```python
from build123d import *

# Parameters (mm, degrees)
BOSS_EXTRUDE1_DEPTH = 3.175
FILLET1_R           = 3.175


with BuildPart() as part:
    # Sketch1 → Boss-Extrude1 (new body)
    with BuildSketch(Plane.XY):
        with BuildLine():
            Line((0, 0), (3.175, 0))
            Line((3.175, 0), (3.175, 6.35))
            Line((3.175, 6.35), (0, 6.35))
            Line((0, 6.35), (0, 12.7))
            Line((0, 12.7), (3.175, 12.7))
            Line((3.175, 12.7), (3.175, 19.05))
            Line((3.175, 19.05), (0, 19.05))
            Line((0, 19.05), (-6.35, 19.05))
            ThreePointArc((-6.35, 19.05), (-9.044076836, 20.165923164), (-10.16, 22.86))
            Line((-10.16, 22.86), (-10.16, 50.8))
            Line((-10.16, 50.8), (-22.86, 50.8))
            Line((-22.86, 50.8), (-22.86, 16.51))
            ThreePointArc((-22.86, 16.51), (-18.024332957, 4.835667043), (-6.35, 0))
            Line((-6.35, 0), (0, 0))
        make_face()
    extrude(amount=BOSS_EXTRUDE1_DEPTH)

    # Fillet1
    fillet1_edges = [part.edges().sort_by_distance(p)[0] for p in [
        (-22.86, 50.8, 1.5875),
        (-10.16, 50.8, 1.5875),
    ]]
    fillet(fillet1_edges, radius=FILLET1_R)


solid = part.part
```
Source: CAD feature listing. Evaluate the final solid. Frame: model axes, mm. A direction names the side the tool comes from. Round coordinates to 2 decimals unless told otherwise and drop trailing zeros. Loops run counter-clockwise (first coordinate to the right, second up) from the corner with the lowest first, then second, coordinate; pieces in that order, holes last. Notation, with made-up numbers: M 16.5,14.25 L 65.5,14.25 A31 cw 65.5,41.25 Z; hole C 27.25,43.25 d10. An arc over 180 degrees is marked long. Use a Markdown table: item, result. Add a question column.
1. Cut plane C-C, the plane x = -3.5. Output: boundary loops of the cut face in (y, z) (3 decimals), and give its area (3 significant figures).
2. Cut plane A-A, the plane x = 1.5. Output: boundary loops of the cut face in (y, z) (3 decimals).
3. Cut plane D-D, the plane y = 45.5. Output: boundary loops of the cut face in (x, z) (3 decimals).
4. Set-up query: faces 1 (the flat face through (0, 9, 2)), 2 (the flat face through (-2, 19.05, 2)), 3 (the flat face through (3.175, 3, 2)). Return all of +Z, -Z, +X, -X, +Y, -Y with unobstructed straight access to the full face (end or side cutting, diameter ignored); none if empty.
5. Cut plane B-B, the plane z = 0.95. Output: boundary loops of the cut face in (x, y) (3 decimals), and give its area (3 significant figures).
6. Ray query, line 1 along Y through (x, z) = (0.5, 1.55); line 2 along Y through (x, z) = (-4.25, 2.5); line 3 along X through (y, z) = (31.5, 1.8). Return the intervals inside material, ascending. Write a range as [from, to].
7. Contact query for flat-ended pins moving along their axis: pin 1 (1.6 mm diameter, centred on y = 33.5, z = 2, fed in from +X); pin 2 (1 mm diameter, centred on y = 8, z = 1.5, fed in from -X); pin 3 (1 mm diameter, centred on x = 2, z = 2, fed in from +Y). Output: stop coordinate, or through.
8. Pull-direction query (Y, two-part tool) for faces 4 (the flat face through (-22.86, 32, 2)), 5 (the flat face through (-2, 0, 2)), 6 (the flat face through (2, 6.35, 2)); classes: +Y half, -Y half, draft (parallel to the pull), parting line (faces both ways), or undercut.
Solution:
| question | item | result |
|---|---|---|
| 1 | outline | M 0,0 L 19.05,0 L 19.05,3.175 L 0,3.175 Z |
| 1 | area | 60.5 mm2 |
| 2 | outline | M 0,0 L 6.35,0 L 6.35,3.175 L 0,3.175 Z; M 12.7,0 L 19.05,0 L 19.05,3.175 L 12.7,3.175 Z |
| 3 | outline | M -22.86,0 L -10.16,0 L -10.16,3.175 L -22.86,3.175 Z |
| 4 | face 1 | +Z, -Z, +X |
| 4 | face 2 | +Z, -Z, +X, +Y |
| 4 | face 3 | +Z, -Z, +X, +Y, -Y |
| 5 | outline | M -22.86,16.51 A16.51 ccw -6.35,0 L 3.175,0 L 3.175,6.35 L 0,6.35 L 0,12.7 L 3.175,12.7 L 3.175,19.05 L -6.35,19.05 A3.81 cw -10.16,22.86 L -10.16,47.625 A3.175 ccw -13.335,50.8 L -19.685,50.8 A3.175 ccw -22.86,47.625 Z |
| 5 | area | 819 mm2 |
| 6 | line 1 | y = [0, 6.35], [12.7, 19.05] |
| 6 | line 2 | y = [0, 19.05] |
| 6 | line 3 | x = [-22.86, -10.16] |
| 7 | pin 1 | stops at x = -10.16 |
| 7 | pin 2 | stops at x = -20.79 |
| 7 | pin 3 | stops at y = 19.05 |
| 8 | face 4 | draft |
| 8 | face 5 | -Y half |
| 8 | face 6 | undercut |
